Design review of the part built by this model. Coordinates are the model's own, in mm. Face numbers are marked on the shaded views. Coordinates: 2 decimals unless noted, no trailing zeros. Write each loop counter-clockwise with the first axis right and the second up, starting at its lowest first coordinate (ties: lowest second). Pieces come first, ordered by that corner, then holes. Notation, with made-up numbers: (41.25, 1) -> (62.25, 1) arc R21 cw to (62.25, 23) -> close; hole circle Ø11 at (81.25, -38). An arc over 180 degrees is marked (long way). Answer in a Markdown table with one row per item. Add a question column.
Item 1: Take a section at A-A, the plane z = 0. Write out the cut boundary in (x, y).
Item 2: Take a section at B-B, the plane x = 6. Write out the cut boundary in (y, z), and give its area (3 significant figures).
Item 3: To check wall thickness, follow line 1 (Y direction, x = 13.75, z = 0); line 2 (X direction, y = 34, z = 7); line 3 (X direction, y = -57, z = 51.5). State the ranges of each line that lie inside material, in increasing order.
Item 4: Draft analysis for pull direction Y (two halves, no side actions). For the marked faces 1, 2 and 3, state which applies: released by +Y, released by -Y, zero draft, split by the parting line, or undercut.
Item 5: Take a section at C-C, the plane x = 42.5. Write out the cut boundary in (y, z).
Item 6: Clearance check with flat-ended pins moving along their axes: P1, Ø1.5, axis at x = 19, y = 19.5, coming from the +Z side; P2, Ø6, axis at x = 20, y = 46.5, coming from the +Z side; P3, Ø12, axis at x = 25.5, z = -6.5, coming from the +Y side. State where each tip first meets the part, or that it passes through.
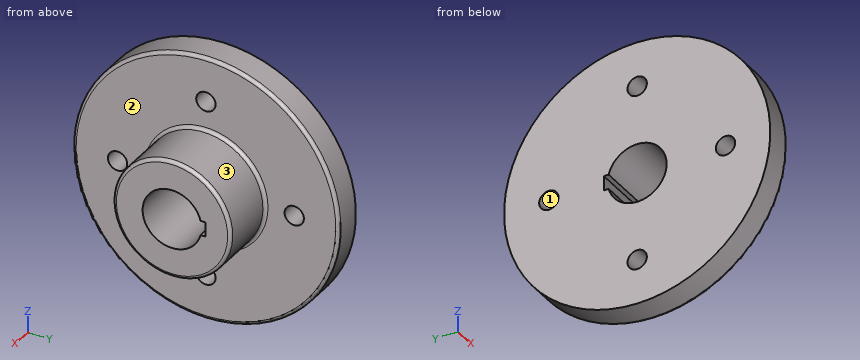
from build123d import *

# Parameters (mm, degrees)
SKETCH1_R           = 82.5
BOSS_EXTRUDE1_DEPTH = 18
SKETCH2_R           = 36.5
BOSS_EXTRUDE2_DEPTH = 36
SKETCH3_R           = 18.25
CUT_EXTRUDE1_DEPTH  = 129.563214023
SKETCH4_R           = 6
CUT_EXTRUDE2_DEPTH  = 129.563214023
FILLET1_R           = 2
SKETCH5_W           = 9
SKETCH5_H           = 3
CUT_EXTRUDE3_DEPTH  = 129.563214023


with BuildPart() as part:
    # Sketch1 → Boss-Extrude1 (new body)
    with BuildSketch(Plane(origin=(0, 0, 0), x_dir=(0, 0, -1), z_dir=(1, 0, 0))):
        Circle(SKETCH1_R)
    extrude(amount=BOSS_EXTRUDE1_DEPTH)

    # Sketch2 → Boss-Extrude2 (add)
    with BuildSketch(Plane(origin=(18, 0, 0), x_dir=(0, 0, -1), z_dir=(1, 0, 0))):
        Circle(SKETCH2_R)
    extrude(amount=BOSS_EXTRUDE2_DEPTH)

    # Sketch3 → Cut-Extrude1 (cut, through all)
    with BuildSketch(Plane.ZY):
        Circle(SKETCH3_R)
    extrude(amount=-CUT_EXTRUDE1_DEPTH, mode=Mode.SUBTRACT)

    # Sketch4 → Cut-Extrude2 (cut, through all)
    with BuildSketch(Plane.ZY):
        with Locations((0, -54.75)):
            Circle(SKETCH4_R)
        with Locations((-54.75, 0)):
            Circle(SKETCH4_R)
        with Locations((0, 54.75)):
            Circle(SKETCH4_R)
        with Locations((54.75, 0)):
            Circle(SKETCH4_R)
    extrude(amount=-CUT_EXTRUDE2_DEPTH, mode=Mode.SUBTRACT)

    # Fillet1
    fillet1_edges = [part.edges().sort_by_distance(p)[0] for p in [
        (18, 0, 82.5),
        (18, 0, 36.5),
        (54, 0, 36.5),
    ]]
    fillet(fillet1_edges, radius=FILLET1_R)

    # Sketch5 → Cut-Extrude3 (cut, through all)
    with BuildSketch(Plane.ZY):
        with Locations((0, 19.186506156)):
            Rectangle(SKETCH5_W, SKETCH5_H)
    extrude(amount=-CUT_EXTRUDE3_DEPTH, mode=Mode.SUBTRACT)


solid = part.part
Answers:
| question | item | result |
|---|---|---|
| 1 | outline | (0, -82.5) -> (16, -82.5) arc R2 ccw to (18, -80.5) -> (18, -60.75) -> (0, -60.75) -> close; (0, -48.75) -> (18, -48.75) -> (18, -38.5) arc R2 cw to (20, -36.5) -> (52, -36.5) arc R2 ccw to (54, -34.5) -> (54, -18.25) -> (0, -18.25) -> close; (0, 20.69) -> (54, 20.69) -> (54, 34.5) arc R2 ccw to (52, 36.5) -> (20, 36.5) arc R2 cw to (18, 38.5) -> (18, 48.75) -> (0, 48.75) -> close; (0, 60.75) -> (18, 60.75) -> (18, 80.5) arc R2 ccw to (16, 82.5) -> (0, 82.5) -> close |
| 2 | outline | circle Ø165 at (0, 0); hole circle Ø12 at (-54.75, 0); hole circle Ø12 at (0, -54.75); hole circle Ø12 at (0, 54.75); hole (17.69, -4.5) -> (20.69, -4.5) -> (20.69, 4.5) -> (17.69, 4.5) arc R18.25 ccw (long way) to start; hole circle Ø12 at (54.75, 0) |
| 2 | area | 19,900 mm^2 |
| 3 | line 1 | y = -82.5 to -60.75, -48.75 to -18.25, 20.69 to 48.75, 60.75 to 82.5 |
| 3 | line 2 | x = 0 to 53.99 |
| 3 | line 3 | x = 0 to 18 |
| 4 | face 1 | undercut |
| 4 | face 2 | zero draft |
| 4 | face 3 | split by the parting line |
| 5 | outline | circle Ø73 at (0, 0); hole (17.69, -4.5) -> (20.69, -4.5) -> (20.69, 4.5) -> (17.69, 4.5) arc R18.25 ccw (long way) to start |
| 6 | P1 | stops at z = 32.13 |
| 6 | P2 | stops at z = 68.46 |
| 6 | P3 | stops at y = 36.5 |
